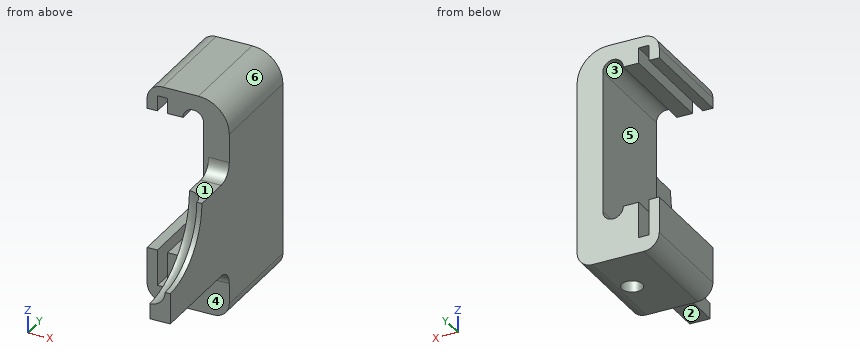
from build123d import *

# Parameters (mm, degrees)
BOSS_EXTRUDE1_DEPTH     = 20
SKETCH3_W               = 12
SKETCH3_H               = 20
BOSS_EXTRUDE2_DEPTH     = 5
FILLET1_R               = 6
FILLET2_R               = 3
SKETCH4_R               = 2
CUT_EXTRUDE1_DEPTH      = 6
SKETCH5_W               = 2
SKETCH5_H               = 20
SKETCH5_W_2             = 3
BOSS_EXTRUDE3_DEPTH     = 4
SKETCH6_W               = 2
SKETCH6_H               = 20
BOSS_EXTRUDE4_DEPTH     = 3
SKETCH7_W               = 2
SKETCH7_H               = 20
BOSS_EXTRUDE5_DEPTH     = 7
FILLET3_R               = 3
SKETCH8_W               = 18
SKETCH8_H               = 22
BOSS_EXTRUDE6_DEPTH     = 5
CUT_EXTRUDE2_DEPTH      = 36.285832851
CUT_EXTRUDE2_DEPTH_BACK = 4
CUT_EXTRUDE3_DEPTH      = 36.285832851
CUT_EXTRUDE3_DEPTH_BACK = 36.285832851
FILLET4_R               = 3
SKETCH11_W              = 18
SKETCH11_H              = 22
CUT_EXTRUDE4_DEPTH      = 1
FILLET5_R               = 3


with BuildPart() as part:
    # Sketch1 → Boss-Extrude1 (new body)
    with BuildSketch(Plane(origin=(0, 0, 0), x_dir=(1, 0, 0), z_dir=(0, 1, 0))):
        with BuildLine():
            Line((0, 15.3), (0, -12.3))
            ThreePointArc((0, -12.3), (-2, -14.3), (-4, -12.3))
            Line((-4, -12.3), (-7, -12.3))
            Line((-7, -12.3), (-7, -17.3))
            Line((-7, -17.3), (5, -17.3))
            Line((5, -17.3), (5, 20.3))
            Line((5, 20.3), (-7, 20.3))
            Line((-7, 20.3), (-7, 15.3))
            Line((-7, 15.3), (-4, 15.3))
            ThreePointArc((-4, 15.3), (-2, 17.3), (0, 15.3))
        make_face()
    extrude(amount=BOSS_EXTRUDE1_DEPTH)

    # Sketch3 → Boss-Extrude2 (add)
    with BuildSketch(Plane(origin=(0, 0, -20.3), x_dir=(-1, 0, 0), z_dir=(0, 0, -1))):
        with Locations((1, 10)):
            Rectangle(SKETCH3_W, SKETCH3_H)
    extrude(amount=BOSS_EXTRUDE2_DEPTH)

    # Fillet1
    fillet1_edges = [part.edges().sort_by_distance(p)[0] for p in [
        (5, 10, 17.3),
    ]]
    fillet(fillet1_edges, radius=FILLET1_R)

    # Fillet2
    fillet2_edges = [part.edges().sort_by_distance(p)[0] for p in [
        (5, 10, -25.3),
    ]]
    fillet(fillet2_edges, radius=FILLET2_R)

    # Sketch4 → Cut-Extrude1 (cut)
    with BuildSketch(Plane(origin=(0, 0, -25.3), x_dir=(-1, 0, 0), z_dir=(0, 0, -1))):
        with Locations((0.5, 10)):
            Circle(SKETCH4_R)
    extrude(amount=-CUT_EXTRUDE1_DEPTH, mode=Mode.SUBTRACT)

    # Sketch5 → Boss-Extrude3 (add)
    with BuildSketch(Plane.ZY.offset(7)):
        with Locations((16.3, 10)):
            Rectangle(SKETCH5_W, SKETCH5_H)
        with Locations((-23.8, 10)):
            Rectangle(SKETCH5_W_2, SKETCH5_H)
    extrude(amount=BOSS_EXTRUDE3_DEPTH)

    # Sketch6 → Boss-Extrude4 (add)
    with BuildSketch(Plane(origin=(0, 0, 15.3), x_dir=(-1, 0, 0), z_dir=(0, 0, -1))):
        with Locations((10, 10)):
            Rectangle(SKETCH6_W, SKETCH6_H)
    extrude(amount=BOSS_EXTRUDE4_DEPTH)

    # Sketch7 → Boss-Extrude5 (add)
    with BuildSketch(Plane.XY.offset(-22.3)):
        with Locations((-10, 10)):
            Rectangle(SKETCH7_W, SKETCH7_H)
    extrude(amount=BOSS_EXTRUDE5_DEPTH)

    # Fillet3
    fillet3_edges = [part.edges().sort_by_distance(p)[0] for p in [
        (-11, 10, 17.3),
        (-11, 10, -25.3),
    ]]
    fillet(fillet3_edges, radius=FILLET3_R)

    # Sketch8 → Boss-Extrude6 (add)
    with BuildSketch(Plane.ZY):
        with Locations((-6.3, -11)):
            Rectangle(SKETCH8_W, SKETCH8_H)
    extrude(amount=-BOSS_EXTRUDE6_DEPTH)

    # Sketch9 → Cut-Extrude2 (cut, two sides: drawn at the far end of the back side and taken through both)
    with BuildSketch(Plane.ZY.offset(-CUT_EXTRUDE2_DEPTH_BACK)):
        with BuildLine():
            Line((2.7, -10.2), (2.7, -7.2))
            ThreePointArc((2.7, -7.2), (-7.835653753, -11.522921748), (-12.298666607, -22))
            Line((-12.298666607, -22), (-9.298333218, -22))
            ThreePointArc((-9.298333218, -22), (-5.714273587, -13.644300146), (2.7, -10.2))
        make_face()
    extrude(amount=CUT_EXTRUDE2_DEPTH + CUT_EXTRUDE2_DEPTH_BACK, mode=Mode.SUBTRACT)

    # Sketch9<3> → Cut-Extrude3 (cut, two sides: drawn at the far end of the back side and taken through both)
    with BuildSketch(Plane.ZY.offset(-CUT_EXTRUDE3_DEPTH_BACK)):
        with BuildLine():
            Line((2.7, -22), (2.7, -10.2))
            ThreePointArc((2.7, -10.2), (-5.714273587, -13.644300146), (-9.298333218, -22))
            Line((-9.298333218, -22), (2.7, -22))
        make_face()
    extrude(amount=CUT_EXTRUDE3_DEPTH + CUT_EXTRUDE3_DEPTH_BACK, mode=Mode.SUBTRACT)

    # Fillet4
    fillet4_edges = [part.edges().sort_by_distance(p)[0] for p in [
        (4, -11.522921748, -7.835653753),
    ]]
    fillet(fillet4_edges, radius=FILLET4_R - 0.0001)  # a hair under: the kernel refuses the full size

    # Sketch11 → Cut-Extrude4 (cut)
    with BuildSketch(Plane.ZY):
        with Locations((-6.3, -11)):
            Rectangle(SKETCH11_W, SKETCH11_H)
    extrude(amount=-CUT_EXTRUDE4_DEPTH, mode=Mode.SUBTRACT)

    # Fillet5
    fillet5_edges = [part.edges().sort_by_distance(p)[0] for p in [
        (3, 0, -15.3),
        (3, 0, 2.7),
    ]]
    fillet(fillet5_edges, radius=FILLET5_R)


solid = part.part
Input: part model. Units: mm. Frame: model coordinates. Face numbers are marked on the shaded views. A direction names the side the tool comes from. Round coordinates to 2 decimals unless told otherwise and drop trailing zeros. Order: outer loops, then holes, each group sorted by start corner. A loop starts at its lowest first (then second) coordinate and runs counter-clockwise, first axis right, second up. Notation, with made-up numbers: (-29, 79) - (-21, 79) arc R30 ccw to (-21, 106) - close; hole circle Ø2 at (62.5, -20). An arc over 180 degrees is marked (long way). Answer as a JSON object with one key per item and string values. Group by question number.
(1) Cut plane D-D (x = 3.25). Return loops of the section in (y, z), then the cut area to 3 significant figures.
(2) Pin query (flat end, axial travel): P1, Ø2, axis at x = 2.5, y = -15, coming from the -Z side; P2, Ø5, axis at y = 4.5, z = -8.5, coming from the -X side; P3, Ø1.6, axis at x = -10.5, y = 8.5, coming from the -Z side. Return the tip coordinate at first contact, or that it passes through.
(3) Cut plane A-A (x = -7.5). Return loops of the section in (y, z).
(4) Material intervals for probe 1 along X at (y, z) = (17.5, -19); probe 2 along X at (y, z) = (17.5, -12); probe 3 along X at (y, z) = (11, 14.5), sorted ascending. Write a range as from..to.
(5) Cut plane B-B (y = 3.5). Return loops of the section in (x, z), then the cut area to 3 significant figures.
(6) Reachability of the marked faces 1, 2 and 3 from +Z, -Z, +X, -X, +Y, -Y: full face, straight path, thin tool, end or side. Return the list, or none.
(7) Cut plane C-C (x = -2). Return loops of the section in (y, z), then the cut area to 3 significant figures.
(8) Draft query along Z for the marked faces 4, 5 and 6. Return one class per face: released by +Z, released by -Z, zero draft, split by the parting line, or undercut.
Here are the results:
{
 "1": {"outline": "(-22, -15.3) - (-3, -15.3) arc R3 cw to (0, -18.3) - (0, -25.03) - (20, -25.03) - (20, 15.54) - (0, 15.54) - (0, 5.7) arc R3 cw to (-3, 2.7) - (-8.22, 2.7) arc R13.98 cw to (-22, -11.28) - close", "area": "1,060 mm^2"},
 "2": {"P1": "stops at z = -15.3", "P2": "stops at x = 0", "P3": "stops at z = -24.77"},
 "3": {"outline": "(0, -25.3) - (20, -25.3) - (20, -22.3) - (0, -22.3) - close; (0, 15.3) - (20, 15.3) - (20, 17.3) - (0, 17.3) - close"},
 "4": {"probe 1": "x = -11..-9, -7..5", "probe 2": "x = 0..5", "probe 3": "x = -10.99..-9, -7..4.08"},
 "5": {"outline": "(-11, -22.3) arc R3 ccw to (-8, -25.3) - (2, -25.3) arc R3 ccw to (5, -22.3) - (5, 11.3) arc R6 ccw to (-1, 17.3) - (-8, 17.3) arc R3 ccw to (-11, 14.3) - (-11, 12.3) - (-9, 12.3) - (-9, 15.3) - (-7, 15.3) - (-7, 12.3) - (-4, 12.3) arc R2 cw to (0, 12.3) - (0, -15.3) arc R2 cw to (-4, -15.3) - (-7, -15.3) - (-7, -22.3) - (-9, -22.3) - (-9, -15.3) - (-11, -15.3) - close", "area": "332 mm^2"},
 "6": {"face 1": "+Z, +X, -X, -Y", "face 2": "-Z, +X, -X, -Y", "face 3": "+Y, -Y"},
 "7": {"outline": "(0, -25.3) - (8.68, -25.3) - (8.68, -19.3) - (11.32, -19.3) - (11.32, -25.3) - (20, -25.3) - (20, -17.3) - (0, -17.3) - close; (0, 14.3) - (20, 14.3) - (20, 17.3) - (0, 17.3) - close", "area": "204 mm^2"},
 "8": {"face 4": "zero draft", "face 5": "undercut", "face 6": "released by +Z"}
}
